Model file for the job. Use its own axes, mm. A direction names the side the tool comes from. Coordinates: 2 decimals unless noted, no trailing zeros. Loops run counter-clockwise (first coordinate to the right, second up) from the corner with the lowest first, then second, coordinate; pieces in that order, holes last. Notation, with made-up numbers: M 55.5,12 L 108.5,12 A20 cw 108.5,22 Z; hole C 1,6 d2. An arc over 180 degrees is marked long. Write item = value, one per line. Start each with the question number.
from build123d import *

# Parameters (mm, degrees)
SKETCH_W      = 61
SKETCH_H      = 11.4
SKETCH_W_2    = 57
SKETCH_H_2    = 7.4
PAD_DEPTH     = 3.5
SKETCH001_W   = 61
SKETCH001_H   = 11.4
PAD001_DEPTH  = 2
CHAMFER_SIZE2 = 1
CHAMFER_SIZE  = 0.25


with BuildPart() as part:
    # Sketch → Pad (new body)
    with BuildSketch(Plane.XY):
        Rectangle(SKETCH_W, SKETCH_H)
        Rectangle(SKETCH_W_2, SKETCH_H_2, mode=Mode.SUBTRACT)
    extrude(amount=PAD_DEPTH)

    # Sketch001 (on Face9 of Pad) → Pad001 (join)
    with BuildSketch(Plane(origin=(0, 0, 0), x_dir=(1, 0, 0), z_dir=(0, 0, -1))):
        Rectangle(SKETCH001_W, SKETCH001_H)
    extrude(amount=PAD001_DEPTH)

    # Chamfer
    chamfer_edges = [part.edges().sort_by_distance(p)[0] for p in [
        (0, 3.7, 3.5),
        (-28.5, 0, 3.5),
        (0, -3.7, 3.5),
        (28.5, 0, 3.5),
    ]]
    chamfer_side = part.faces().sort_by_distance((29.879439, 0, 3.5))[0]
    chamfer(chamfer_edges, length=CHAMFER_SIZE, length2=CHAMFER_SIZE2, reference=chamfer_side)


solid = part.part
Item 1: Pull direction Y, two halves, no side cores. Call faces 3 (the flat face through (0, 3.7, 1)), 4 (the flat face through (0, 5.7, 1)), 5 (the flat face through (-0.1, 4.2, 3.5)): +Y half, -Y half, draft (parallel to the pull), parting line (faces both ways), or undercut.
Item 2: Cut at C-C (y = -1.25). Give the cut face in (x, z).
Item 3: Probe L1, parallel to Y at x = 4, z = 2.15; L2, parallel to X at y = 1.5, z = 2.25; L3, parallel to Z at x = 16.5, y = -1.25. List the from-to ranges inside material, lowest first.
Item 4: Cut at A-A (z = 0.9). Give the cut face in (x, y).
Item 5: 3-axis set-ups, long thin cutter, end or side, ignore diameter. For faces 1 (the flat face through (30.5, 0, 1)), 2 (the flat face through (-0.402, -3.823, 2.993)): which of +Z, -Z, +X, -X, +Y, -Y reach the whole face in a straight line?
Item 6: Pin check, flat tip, straight feed: pin 1 Ø1.5 at (x, y) = (3.5, -2) entering from +Z. Stop position of the tip, or through.
Item 7: Cut at B-B (x = 18). Give the cut face in (y, z), plus the area to 4 significant figures.
Reported:
q1.face_3 = undercut
q1.face_4 = +Y half
q1.face_5 = draft
q2.outline = M -30.5,-2 L 30.5,-2 L 30.5,3.5 L 28.75,3.5 L 28.5,2.5 L 28.5,0 L -28.5,0 L -28.5,2.5 L -28.75,3.5 L -30.5,3.5 Z
q3.L1 = -5.7 to -3.7, 3.7 to 5.7
q3.L2 = -30.5 to -28.5, 28.5 to 30.5
q3.L3 = -2 to 0
q4.outline = M -30.5,-5.7 L 30.5,-5.7 L 30.5,5.7 L -30.5,5.7 Z; hole M -28.5,-3.7 L 28.5,-3.7 L 28.5,3.7 L -28.5,3.7 Z
q5.face_1 = +Z, -Z, +X, +Y, -Y
q5.face_2 = +Z
q6.pin_1 = 0
q7.outline = M -5.7,-2 L 5.7,-2 L 5.7,3.5 L 3.95,3.5 L 3.7,2.5 L 3.7,0 L -3.7,0 L -3.7,2.5 L -3.95,3.5 L -5.7,3.5 Z
q7.area = 36.55 mm^2
